Autodesk Inventor part; units mm, degrees
ref_plane "Начальная плоскость" through (0, 0, 10) normal (0, 0, 1) x (1, 0, 0)
ref_plane "Конечная плоскость" through (0, 0, 40) normal (0, 0, 1) x (1, 0, 0)
ref_plane "РабПлоскость6" through (0, 0, 40) normal (0, 0, 1) x (1, 0, 0)
ref_plane "Начальная плоскость" through (0, 0, 10) normal (0, 0, 1) x (1, 0, 0)
ref_plane "Конечная плоскость" through (0, 0, 40) normal (0, 0, 1) x (1, 0, 0)
sketch "Эскиз" plane through (0, 0, 0) normal (0, 0, 1) x (1, 0, 0)
  line L0 (-14.4349, 0) -> (14.4349, 0)
  line L1 (0, -14) -> (0, 14)
  line L2 (0, 0) -> (7.5, 7.5) construction
  circle A0 centre (7.5, 7.5) radius 1.65 construction
  line L3 (5.85, 9.15) -> (9.15, 9.15)
  line L4 (9.15, 9.15) -> (9.15, 5.85)
  line L5 (9.15, 5.85) -> (5.85, 5.85)
  line L6 (5.85, 5.85) -> (5.85, 9.15)
  line L7 (3.235, 8.1636) -> (4.72, 9.9636)
  line L8 (4.7971, 10) -> (8.5, 10)
  line L9 (3.3121, 8) -> (4.95, 8)
  line L10 (4.95, 8) -> (4.95, 5.7985)
  line L11 (4.95, 5.7985) -> (2.6515, 3.5)
  line L12 (0, 3.5) -> (2.6515, 3.5)
  circle A1 centre (0, 0) radius 2.5
  line L13 (8.1636, 3.235) -> (9.9636, 4.72)
  line L14 (10, 4.7971) -> (10, 8.5)
  line L15 (8, 3.3121) -> (8, 4.95)
  line L16 (8, 4.95) -> (5.7985, 4.95)
  line L17 (5.7985, 4.95) -> (3.5, 2.6515)
  line L18 (3.5, 0) -> (3.5, 2.6515)
  arc A2 (10, 8.5) -> (8.5, 10) centre (8.5, 8.5) ccw
  line L19 (0, 0) -> (-7.5, 7.5) construction
  circle A3 centre (-7.5, 7.5) radius 1.65 construction
  line L20 (-5.85, 9.15) -> (-9.15, 9.15)
  line L21 (-9.15, 9.15) -> (-9.15, 5.85)
  line L22 (-9.15, 5.85) -> (-5.85, 5.85)
  line L23 (-5.85, 5.85) -> (-5.85, 9.15)
  line L24 (-3.235, 8.1636) -> (-4.72, 9.9636)
  line L25 (-4.7971, 10) -> (-8.5, 10)
  line L26 (-3.3121, 8) -> (-4.95, 8)
  line L27 (-4.95, 8) -> (-4.95, 5.7985)
  line L28 (-4.95, 5.7985) -> (-2.6515, 3.5)
  line L29 (0, 3.5) -> (-2.6515, 3.5)
  line L30 (-3.5, 0) -> (-3.5, 2.6515)
  line L31 (-5.7985, 4.95) -> (-3.5, 2.6515)
  line L32 (-8, 4.95) -> (-5.7985, 4.95)
  line L33 (-8, 3.3121) -> (-8, 4.95)
  line L34 (-8.1636, 3.235) -> (-9.9636, 4.72)
  line L35 (-10, 4.7971) -> (-10, 8.5)
  arc A4 (-8.5, 10) -> (-10, 8.5) centre (-8.5, 8.5) ccw
  line L36 (0, 14) -> (0, -14)
  line L37 (0, 0) -> (7.5, -7.5) construction
  circle A5 centre (7.5, -7.5) radius 1.65 construction
  line L38 (5.85, -9.15) -> (9.15, -9.15)
  line L39 (9.15, -9.15) -> (9.15, -5.85)
  line L40 (9.15, -5.85) -> (5.85, -5.85)
  line L41 (5.85, -5.85) -> (5.85, -9.15)
  line L42 (3.235, -8.1636) -> (4.72, -9.9636)
  line L43 (4.7971, -10) -> (8.5, -10)
  line L44 (3.3121, -8) -> (4.95, -8)
  line L45 (4.95, -8) -> (4.95, -5.7985)
  line L46 (4.95, -5.7985) -> (2.6515, -3.5)
  line L47 (0, -3.5) -> (2.6515, -3.5)
  line L48 (3.5, 0) -> (3.5, -2.6515)
  line L49 (5.7985, -4.95) -> (3.5, -2.6515)
  line L50 (8, -4.95) -> (5.7985, -4.95)
  line L51 (8, -3.3121) -> (8, -4.95)
  line L52 (8.1636, -3.235) -> (9.9636, -4.72)
  line L53 (10, -4.7971) -> (10, -8.5)
  arc A6 (8.5, -10) -> (10, -8.5) centre (8.5, -8.5) ccw
  line L54 (0, 0) -> (-7.5, -7.5) construction
  line L55 (-4.95, -8) -> (-4.95, -5.7985)
  line L56 (-3.3121, -8) -> (-4.95, -8)
  line L57 (-5.7985, -4.95) -> (-3.5, -2.6515)
  line L58 (-4.95, -5.7985) -> (-2.6515, -3.5)
  line L59 (-3.5, 0) -> (-3.5, -2.6515)
  line L60 (0, -3.5) -> (-2.6515, -3.5)
  circle A7 centre (-7.5, -7.5) radius 1.65 construction
  line L61 (-5.85, -5.85) -> (-5.85, -9.15)
  line L62 (-5.85, -9.15) -> (-9.15, -9.15)
  line L63 (-9.15, -9.15) -> (-9.15, -5.85)
  line L64 (-9.15, -5.85) -> (-5.85, -5.85)
  line L65 (-3.235, -8.1636) -> (-4.72, -9.9636)
  line L66 (-8, -4.95) -> (-5.7985, -4.95)
  line L67 (-8, -3.3121) -> (-8, -4.95)
  line L68 (-8.1636, -3.235) -> (-9.9636, -4.72)
  line L69 (-4.7971, -10) -> (-8.5, -10)
  line L70 (-10, -4.7971) -> (-10, -8.5)
  arc A8 (-10, -8.5) -> (-8.5, -10) centre (-8.5, -8.5) ccw
  arc A9 (3.235, 8.1636) -> (3.3121, 8) centre (3.3121, 8.1) ccw
  arc A10 (4.7971, 10) -> (4.72, 9.9636) centre (4.7971, 9.9) ccw
  arc A11 (8, 3.3121) -> (8.1636, 3.235) centre (8.1, 3.3121) ccw
  arc A12 (9.9636, 4.72) -> (10, 4.7971) centre (9.9, 4.7971) ccw
  arc A13 (-3.3121, 8) -> (-3.235, 8.1636) centre (-3.3121, 8.1) ccw
  arc A14 (-4.72, 9.9636) -> (-4.7971, 10) centre (-4.7971, 9.9) ccw
  arc A15 (-8.1636, 3.235) -> (-8, 3.3121) centre (-8.1, 3.3121) ccw
  arc A16 (-10, 4.7971) -> (-9.9636, 4.72) centre (-9.9, 4.7971) ccw
  arc A17 (-8, -3.3121) -> (-8.1636, -3.235) centre (-8.1, -3.3121) ccw
  arc A18 (-9.9636, -4.72) -> (-10, -4.7971) centre (-9.9, -4.7971) ccw
  arc A19 (-3.235, -8.1636) -> (-3.3121, -8) centre (-3.3121, -8.1) ccw
  arc A20 (-4.7971, -10) -> (-4.72, -9.9636) centre (-4.7971, -9.9) ccw
  arc A21 (4.72, -9.9636) -> (4.7971, -10) centre (4.7971, -9.9) ccw
  arc A22 (3.3121, -8) -> (3.235, -8.1636) centre (3.3121, -8.1) ccw
  arc A23 (8.1636, -3.235) -> (8, -3.3121) centre (8.1, -3.3121) ccw
  arc A24 (10, -4.7971) -> (9.9636, -4.72) centre (9.9, -4.7971) ccw
  point P0 (3.1, 8)
  point P1 (4.75, 10)
  point P2 (7.5, 9.15)
  point P3 (8, 3.1)
  point P4 (10, 4.75)
  point P5 (7.5, 5.85)
  point P6 (9.15, 7.5)
  point P7 (-3.1, 8)
  point P8 (-4.75, 10)
  point P9 (-7.5, 9.15)
  point P10 (-8, 3.1)
  point P11 (-10, 4.75)
  point P12 (-7.5, 5.85)
  point P13 (-9.15, 7.5)
  point P14 (3.1, -8)
  point P15 (4.75, -10)
  point P16 (7.5, -9.15)
  point P17 (8, -3.1)
  point P18 (10, -4.75)
  point P19 (7.5, -5.85)
  point P20 (9.15, -7.5)
  point P21 (-3.1, -8)
  point P22 (-7.5, -5.85)
  point P23 (-7.5, -9.15)
  point P24 (-9.15, -7.5)
  point P25 (-4.75, -10)
  point P26 (-8, -3.1)
  point P27 (-10, -4.75)
  dimension "d0" = 45
  dimension "d1" = 3.3
  dimension "d2" = 1.5
  dimension "d3" = 1.2
  dimension "d4" = 5
  dimension "d5" = 6.5
  dimension "d6" = 15
  dimension "d7" = 20
  dimension "d8" = 9.9
  dimension "d9" = 9.5
  dimension "d10" = 6.2
  dimension "d11" = 2
  dimension "d18" = 0.1
  dimension "d19" = 0.1
extrude "Тело" add sketch "Эскиз" along normal up to surface (30 mm away) from surface at 10 contours A1 L1 L12 L11 L10 L9 A9 L7 A10 L8 A2 L14 A12 L13 A11 L15 L16 L17 L18 L0 | L0 L48 L49 L50 L51 A23 L52 A24 L53 A6 L43 A21 L42 A22 L44 L45 L46 L47 L1 A1 | A1 L0 L30 L31 L32 L33 A15 L34 A16 L35 A4 L25 A14 L24 A13 L26 L27 L28 L29 L1 | L1 L60 L58 L55 L56 A19 L65 A20 L69 A8 L70 A18 L68 A17 L67 L66 L57 L59 L0 A1
sketch "Эскиз2" plane through (0, 0, 0) normal (0, 0, 1) x (1, 0, 0)
  line L0 (0, 0) -> (10, 0)
ref_plane "РабПлоскость3" through (0, 0, 0) normal (0, -1, 0) x (1, 0, 0)
sketch "Эскиз3" plane through (0, 0, 0) normal (0, -1, 0) x (1, 0, 0)
  line L0 (-2, 10) -> (12, 10)
  line L1 (-2, 40) -> (12, 40)
  dimension "d25" = 30
ref_plane "РабПлоскость6" through (0, 0, 40) normal (0, 0, 1) x (1, 0, 0)
split "Разделение3" plane through (0, 0, 40) removes the side toward (0, 0, 1)
ref_plane "РабПлоскость7" through (0, 300, 10) normal (0, 0, -1) x (-1, 0, 0)
split "Разделение4" plane through (0, 300, 10) removes the side toward (0, 0, -1)
properties part number "короткая палка"
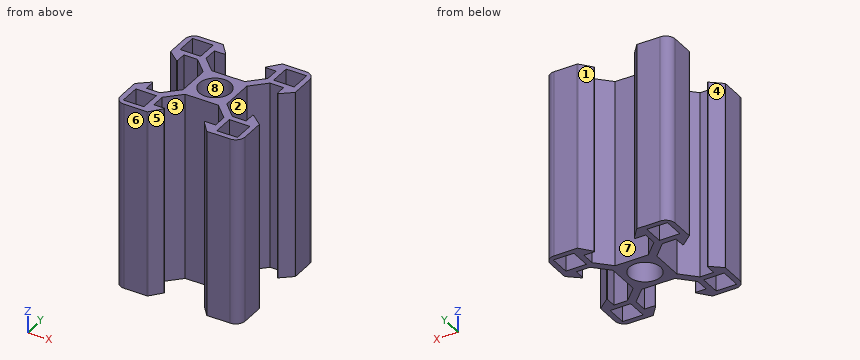
Geometry check sheet. Reference: the model listing, model coordinates, mm. Face numbers are marked on the shaded views. A direction names the side the tool comes from. Round coordinates to 2 decimals unless told otherwise and drop trailing zeros. Loops run counter-clockwise (first coordinate to the right, second up) from the corner with the lowest first, then second, coordinate; pieces in that order, holes last.
Item 1: Mould release check, pull along Y, two halves, no side actions. Record for the marked faces 6, 7 and 8: pulls with the +Y half, pulls with the -Y half, needs draft (parallel to the pull), parting line crosses it, or undercut.
Item 2: Gauge pin test, flat ends, axial feed: pin 1 (0.5 mm diameter, centred on y = -4, z = 19, fed in from -X); pin 2 (3 mm diameter, centred on x = 3, z = 18.5, fed in from +Y); pin 3 (4 mm diameter, centred on y = 0.5, z = 22.5, fed in from +X). Record the tip position at first contact, or that the pin passes through.
Item 3: Cross-section at C-C on y = -7. Record the boundary of the cut face in (x, z).
Item 4: Cross-section at D-D on z = 30.75. Count the separate pieces of the cut face and the enclosed holes in it, then the cut area to 3 significant figures.
Item 5: Cross-section at A-A on x = 0. Record the boundary of the cut face in (y, z), then the cut area to 3 significant figures.
Item 6: Access from +Z, -Z, +X, -X, +Y, -Y to the whole of each face (thin tool, end or side, straight path). Record for the marked faces 1, 2, 3, 4 and 5.
Item 7: Thickness scan on line 1 (X direction, y = -7.5, z = 13.25); line 2 (Y direction, x = 0, z = 21.25). Record the ranges inside material, lowest first.
Answer sheet:
1. face 6: pulls with the -Y half
1. face 7: pulls with the +Y half
1. face 8: undercut
2. pin 1: stops at x = -9.39
2. pin 2: stops at y = 9.7
2. pin 3: stops at x = 3.5
3. outline: (-10, 10) - (-9.15, 10) - (-9.15, 40) - (-10, 40) - close; (-5.85, 10) - (-4.95, 10) - (-4.95, 40) - (-5.85, 40) - close; (4.95, 10) - (5.85, 10) - (5.85, 40) - (4.95, 40) - close; (9.15, 10) - (10, 10) - (10, 40) - (9.15, 40) - close
4. separate pieces: 1
4. enclosed holes: 5
4. area: 115 mm2
5. outline: (-3.5, 10) - (-2.5, 10) - (-2.5, 40) - (-3.5, 40) - close; (2.5, 10) - (3.5, 10) - (3.5, 40) - (2.5, 40) - close
5. area: 60.0 mm2
6. face 1: +Z, -Z, +Y
6. face 2: +Z, -Z, +X
6. face 3: +Z, -Z
6. face 4: +Z, -Z, -X
6. face 5: +Z, -Z, -Y
7. line 1: x = -10 to -9.15, -5.85 to -4.95, 4.95 to 5.85, 9.15 to 10
7. line 2: y = -3.5 to -2.5, 2.5 to 3.5
